```python
from build123d import *

# Parameters (mm, degrees)
SKETCH_1_R      = 5
SKETCH_1_R_2    = 1.075
SKETCH_1_R_3    = 1.575
SKETCH_1_W      = 5
SKETCH_1_H      = 15
SKETCH_1_H_2    = 12.5
EXTRUDE_1_DEPTH = 5
FILLET_1_R      = 5


with BuildPart() as part:
    # 草图1 → 凸台-拉伸1 (new body)
    with BuildSketch(Plane(origin=(0, 0, 0), x_dir=(1, 0, 0), z_dir=(0, 1, 0))):
        Polygon((52.8, -28.197121602), (-52.8, -28.197121602), (-52.8, 46.802878398), (-33.230116948, 46.802878398), (-22.5, 24.802878398), (22.5, 24.802878398), (33.230116948, 46.802878398), (52.8, 46.802878398), align=None)
        with Locations(Location((0, 0, 0), (0, 0, 270))):
            Circle(SKETCH_1_R, mode=Mode.SUBTRACT)
        with Locations(Location((-13.525, 0, 0), (0, 0, 270))):
            Circle(SKETCH_1_R_2, mode=Mode.SUBTRACT)
        with Locations(Location((-10.475, 0, 0), (0, 0, 270))):
            Circle(SKETCH_1_R_2, mode=Mode.SUBTRACT)
        with Locations(Location((-7.425, 0, 0), (0, 0, 270))):
            Circle(SKETCH_1_R_2, mode=Mode.SUBTRACT)
        with Locations(Location((-6.7625, 11.712993586, 0), (0, 0, 270))):
            Circle(SKETCH_1_R_2, mode=Mode.SUBTRACT)
        with Locations(Location((-5.2375, 9.071616105, 0), (0, 0, 270))):
            Circle(SKETCH_1_R_2, mode=Mode.SUBTRACT)
        with Locations(Location((-3.7125, 6.430238623, 0), (0, 0, 270))):
            Circle(SKETCH_1_R_2, mode=Mode.SUBTRACT)
        with Locations(Location((6.7625, 11.712993586, 0), (0, 0, 270))):
            Circle(SKETCH_1_R_2, mode=Mode.SUBTRACT)
        with Locations(Location((5.2375, 9.071616105, 0), (0, 0, 270))):
            Circle(SKETCH_1_R_2, mode=Mode.SUBTRACT)
        with Locations(Location((3.7125, 6.430238623, 0), (0, 0, 270))):
            Circle(SKETCH_1_R_2, mode=Mode.SUBTRACT)
        with Locations(Location((13.525, 0, 0), (0, 0, 270))):
            Circle(SKETCH_1_R_2, mode=Mode.SUBTRACT)
        with Locations(Location((10.475, 0, 0), (0, 0, 270))):
            Circle(SKETCH_1_R_2, mode=Mode.SUBTRACT)
        with Locations(Location((7.425, 0, 0), (0, 0, 270))):
            Circle(SKETCH_1_R_2, mode=Mode.SUBTRACT)
        with Locations(Location((6.7625, -11.712993586, 0), (0, 0, 270))):
            Circle(SKETCH_1_R_2, mode=Mode.SUBTRACT)
        with Locations(Location((5.2375, -9.071616105, 0), (0, 0, 270))):
            Circle(SKETCH_1_R_2, mode=Mode.SUBTRACT)
        with Locations(Location((3.7125, -6.430238623, 0), (0, 0, 270))):
            Circle(SKETCH_1_R_2, mode=Mode.SUBTRACT)
        with Locations(Location((-6.7625, -11.712993586, 0), (0, 0, 270))):
            Circle(SKETCH_1_R_2, mode=Mode.SUBTRACT)
        with Locations(Location((-5.2375, -9.071616105, 0), (0, 0, 270))):
            Circle(SKETCH_1_R_2, mode=Mode.SUBTRACT)
        with Locations(Location((-3.7125, -6.430238623, 0), (0, 0, 270))):
            Circle(SKETCH_1_R_2, mode=Mode.SUBTRACT)
        with Locations(Location((-35, -20, 0), (0, 0, 270))):
            Circle(SKETCH_1_R_3, mode=Mode.SUBTRACT)
        with Locations(Location((-35, 40, 0), (0, 0, 270))):
            Circle(SKETCH_1_R_3, mode=Mode.SUBTRACT)
        with Locations(Location((35, 40, 0), (0, 0, 90))):
            Circle(SKETCH_1_R_3, mode=Mode.SUBTRACT)
        with Locations(Location((35, -20, 0), (0, 0, 90))):
            Circle(SKETCH_1_R_3, mode=Mode.SUBTRACT)
        with Locations((-43.8, 35.802878398)):
            Rectangle(SKETCH_1_W, SKETCH_1_H, mode=Mode.SUBTRACT)
        with Locations((-43.8, 10.802878398)):
            Rectangle(SKETCH_1_W, SKETCH_1_H_2, mode=Mode.SUBTRACT)
        with Locations((-43.8, -14.197121602)):
            Rectangle(SKETCH_1_W, SKETCH_1_H, mode=Mode.SUBTRACT)
        with Locations((43.8, -14.197121602)):
            Rectangle(SKETCH_1_W, SKETCH_1_H, mode=Mode.SUBTRACT)
        with Locations((43.8, 10.802878398)):
            Rectangle(SKETCH_1_W, SKETCH_1_H_2, mode=Mode.SUBTRACT)
        with Locations((43.8, 35.802878398)):
            Rectangle(SKETCH_1_W, SKETCH_1_H, mode=Mode.SUBTRACT)
    extrude(amount=EXTRUDE_1_DEPTH)

    # 圆角1
    fillet_1_edges = [part.edges().sort_by_distance(p)[0] for p in [
        (52.8, 2.5, -46.802878398),
        (52.8, 2.5, 28.197121602),
        (-52.8, 2.5, 28.197121602),
        (-52.8, 2.5, -46.802878398),
    ]]
    fillet(fillet_1_edges, radius=FILLET_1_R)


solid = part.part
```
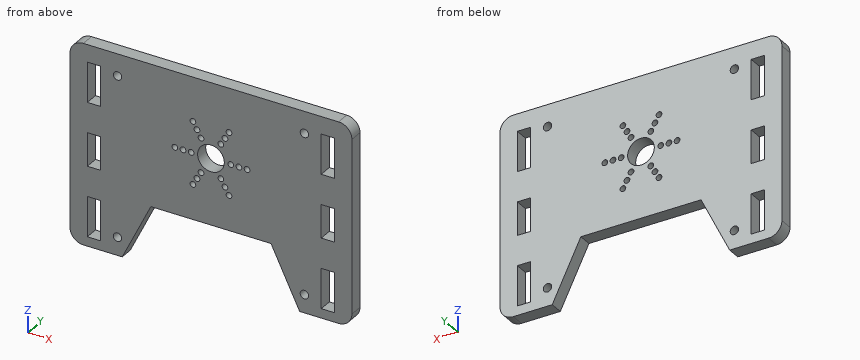
The model under review builds one solid part; all positions refer to its coordinate system, in mm. Give positions to 0.01 mm unless a question says otherwise; leave off trailing zeros. Loops run counter-clockwise (first coordinate to the right, second up) from the corner with the lowest first, then second, coordinate; pieces in that order, holes last. Notation, with made-up numbers: (-2.5, -33.5) - (47.5, -33.5) arc R15 ccw to (47.5, -13.5) - close; hole circle Ø1 at (19.5, 34.5). An arc over 180 degrees is marked (long way). Answer as a JSON object with one key per item and string values.
Q1. Add section A-A on z = 20. State the section outline as (x, y) points (3 decimals), plus the area to 4 significant figures.
Worked out:
{"outline": "(-52.8, 0) - (-46.3, 0) - (-46.3, 5) - (-52.8, 5) - close; (-41.3, 0) - (-36.575, 0) - (-36.575, 5) - (-41.3, 5) - close; (-33.425, 0) - (33.425, 0) - (33.425, 5) - (-33.425, 5) - close; (36.575, 0) - (41.3, 0) - (41.3, 5) - (36.575, 5) - close; (46.3, 0) - (52.8, 0) - (52.8, 5) - (46.3, 5) - close", "area": "446.5 mm^2"}
Q2. Add section B-B on x = -35. State the section outline as (y, z) points (3 decimals), plus the area to 4 significant figures.
Worked out:
{"outline": "(0, -46.803) - (5, -46.803) - (5, -41.575) - (0, -41.575) - close; (0, -38.425) - (5, -38.425) - (5, 18.425) - (0, 18.425) - close; (0, 21.575) - (5, 21.575) - (5, 28.197) - (0, 28.197) - close", "area": "343.5 mm^2"}
Q3. Add section C-C on z = 0. Count the separate pieces of the cut face and the enclosed holes in it, plus the area to 4 significant figures.
Worked out:
{"separate pieces": "8", "enclosed holes": "0", "area": "413.5 mm^2"}
Q4. Insertion check: pin 1 (3 mm diameter, centred on x = 10.5, y = 1, fed in from -Z). The pin has a flat end and moves straight along its axis. Give the tip position at first contact, or say it passes through.
Worked out:
{"pin 1": "stops at z = -24.8"}
Q5. To check wall thickness, follow line 1 along X through (y, z) = (2.7, -9); line 2 along Z through (x, y) = (45, 4.3); line 3 along X through (y, z) = (0.4, -10). State the ranges of each line that lie inside material, in increasing order.
Worked out:
{"line 1": "x = -52.8 to -46.3, -41.3 to -6.31, -4.16 to 4.16, 6.31 to 41.3, 46.3 to 52.8", "line 2": "z = -46.8 to -43.3, -28.3 to -17.05, -4.55 to 6.7, 21.7 to 28.2", "line 3": "x = -52.8 to -46.3, -41.3 to -5.78, -4.7 to 4.7, 5.78 to 41.3, 46.3 to 52.8"}
Q6. Add section D-D on z = -40. State the section outline as (x, y) points (3 decimals), plus the area to 3 significant figures.
Worked out:
{"outline": "(-52.8, 0) - (-46.3, 0) - (-46.3, 5) - (-52.8, 5) - close; (-41.3, 0) - (-36.575, 0) - (-36.575, 5) - (-41.3, 5) - close; (-33.425, 0) - (-29.912, 0) - (-29.912, 5) - (-33.425, 5) - close; (29.912, 0) - (33.425, 0) - (33.425, 5) - (29.912, 5) - close; (36.575, 0) - (41.3, 0) - (41.3, 5) - (36.575, 5) - close; (46.3, 0) - (52.8, 0) - (52.8, 5) - (46.3, 5) - close", "area": "147 mm^2"}
